Design review of the part built by this model. Coordinates are the model's own, in mm. Round coordinates to 2 decimals unless told otherwise and drop trailing zeros. Loops run counter-clockwise (first coordinate to the right, second up) from the corner with the lowest first, then second, coordinate; pieces in that order, holes last. Notation, with made-up numbers: (-1.5, 32.5) - (17.5, 32.5) arc R18 cw to (17.5, 38.5) - close; hole circle Ø1 at (78, 21). An arc over 180 degrees is marked (long way). Use one line per item in the form item = value. Start each with the question number.
(1) Wall thickness on probe 1 along Z at (x, y) = (0, -51.5); probe 2 along Z at (x, y) = (2, -33); probe 3 along X at (y, z) = (-49, 43.5): over which ranges is each line inside the solid? List them lowest first. Write a range as [from, to].
(2) We need section A-A, the plane x = 0. Write out the cut boundary in (y, z), then the cut area to 3 significant figures.
(3) We need section C-C, the plane y = -54. Write out the cut boundary in (x, z), then the cut area to 3 significant figures.
(4) We need section B-B, the plane y = -31.5. Write out the cut boundary in (x, z), then the cut area to 3 significant figures.
(5) For pin 1 (6 mm diameter, centred on y = -30, z = 31, fed in from +X); pin 2 (8 mm diameter, centred on x = -4, y = -35, fed in from -Z); pin 3 (1.5 mm diameter, centred on x = 1, z = 39.5, fed in from +Y); pin 4 (12 mm diameter, centred on x = 8, y = -53.5, fed in from +Z), all flat-tipped, find the tip position at first contact; note any pin that passes through.
(6) The part is to be moulded in two halves that separate along Z. For faces 1 (the flat face through (0, -18.716, 44)), 2 (the conical face through (-0.43, -44.47, 31.25)), 3 (the cylindrical face through (1.54, -44.47, 43.4)), say which applies: released by +Z, released by -Z, zero draft, split by the parting line, or undercut.
from build123d import *

# Parameters (mm, degrees)
F0_R     = 12.7
F1_DEPTH = 63.5
F3_D     = 5.7404
F3_DEPTH = 63.5
F7_D     = 5.7404
F7_DEPTH = 50.8


with BuildPart() as f1:
    # F0 (on Front) → F1 (new body)
    with BuildSketch(Plane.XZ):
        Circle(F0_R)
    extrude(amount=F1_DEPTH)

    # F3
    with Locations(Plane(origin=(0, 0, 0), x_dir=(1, 0, 0), z_dir=(0, 1, 0))):
        with Locations((0, 0)):
            Hole(F3_D / 2, depth=F3_DEPTH)


with BuildPart() as f5:
    # F4 (on Right) → F5 (revolve)
    with BuildSketch(Plane.YZ):
        Polygon((-69.515724, 40.979306), (-18.715724, 40.979306), (-18.715724, 53.679306), (-69.515724, 47.837306), align=None)
    revolve(axis=Axis((0, -44.115724, 40.979306), (0, -1, 0)))

    # F7
    with Locations(Plane(origin=(0, -18.715724, 0), x_dir=(-1, 0, 0), z_dir=(0, 1, 0))):
        with Locations((0, 40.979306)):
            Hole(F7_D / 2, depth=F7_DEPTH)


solid = f5.part
Data:
q1.probe_1 = [32.05, 38.11], [43.85, 49.91]
q1.probe_2 = [30.1, 38.92], [43.04, 51.85]
q1.probe_3 = [-8.87, -1.37], [1.37, 8.87]
q2.outline = (-69.52, 34.12) - (-18.72, 28.28) - (-18.72, 38.11) - (-69.52, 38.11) - close; (-69.52, 43.85) - (-18.72, 43.85) - (-18.72, 53.68) - (-69.52, 47.84) - close
q2.area = 702 mm^2
q3.outline = circle Ø17.28 at (0, 40.98); hole circle Ø5.74 at (0, 40.98)
q3.area = 209 mm^2
q4.outline = circle Ø22.46 at (0, 40.98); hole circle Ø5.74 at (0, 40.98)
q4.area = 370 mm^2
q5.pin_1 = 9.06
q5.pin_2 = 29.89
q5.pin_3 = through
q5.pin_4 = 49.6
q6.face_1 = zero draft
q6.face_2 = split by the parting line
q6.face_3 = undercut
